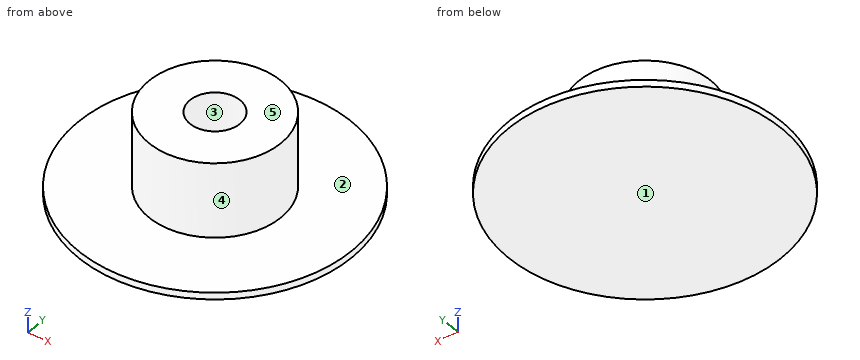
```python
from build123d import *

# Parameters (mm, degrees)
SKETCH1_R           = 30
BOSS_EXTRUDE1_DEPTH = 1.5
SKETCH2_R           = 14.5
SKETCH2_R_2         = 5.5
EXTRUDE_THIN1_DEPTH = 18


with BuildPart() as part:
    # Sketch1 → Boss-Extrude1 (new body)
    with BuildSketch(Plane.XY):
        Circle(SKETCH1_R)
    extrude(amount=BOSS_EXTRUDE1_DEPTH)

    # Sketch2 → Extrude-Thin1 (add)
    with BuildSketch(Plane.XY):
        Circle(SKETCH2_R)
        Circle(SKETCH2_R_2, mode=Mode.SUBTRACT)
    extrude(amount=EXTRUDE_THIN1_DEPTH)


solid = part.part
```
Verification items for the finished model (mm, model axes). Face numbers are marked on the shaded views. A direction names the side the tool comes from. Coordinates: 2 decimals unless noted, no trailing zeros. Loops run counter-clockwise (first coordinate to the right, second up) from the corner with the lowest first, then second, coordinate; pieces in that order, holes last. Notation, with made-up numbers: (-3, 25) -> (41, 25) arc R26 ccw to (41, 54) -> close; hole circle Ø2 at (57.5, -39). An arc over 180 degrees is marked (long way). Put each result on its own line as item: value.
1. Gauge pin test, flat ends, axial feed: P1, Ø10, axis at x = 5, z = 15.5, coming from the -Y side; P2, Ø2, axis at x = 18, y = -12.5, coming from the -Z side; P3, Ø8, axis at x = 3.5, z = 15.5, coming from the +Y side; P4, Ø1.5, axis at x = 2.5, z = 15, coming from the +Y side. Record the tip position at first contact, or that the pin passes through.
Result set:
P1: stops at y = -14.5
P2: stops at z = 0
P3: stops at y = 14.5
P4: stops at y = 14.39
2. Section check A-A, the plane y = 0. Record the boundary of the cut face in (x, z), then the cut area to 3 significant figures.
Result set:
outline: (-30, 0) -> (30, 0) -> (30, 1.5) -> (14.5, 1.5) -> (14.5, 18) -> (5.5, 18) -> (5.5, 1.5) -> (-5.5, 1.5) -> (-5.5, 18) -> (-14.5, 18) -> (-14.5, 1.5) -> (-30, 1.5) -> close
area: 387 mm^2
3. Section check C-C, the plane z = 14.25. Record the boundary of the cut face in (x, y).
Result set:
outline: circle Ø29 at (0, 0); hole circle Ø11 at (0, 0)
4. Mould release check, pull along Y, two halves, no side actions. Record for the marked faces 3, 4 and 5: pulls with the +Y half, pulls with the -Y half, needs draft (parallel to the pull), parting line crosses it, or undercut.
Result set:
face 3: undercut
face 4: parting line crosses it
face 5: needs draft
5. Thickness scan on line 1 (Y direction, x = 0, z = 5.75); line 2 (Z direction, x = -10, y = -18). Record the ranges inside material, lowest first.
Result set:
line 1: y = -14.5 to -5.5, 5.5 to 14.5
line 2: z = 0 to 1.5
6. Tool access check on the marked faces 1 and 2. Record the directions out of +Z, -Z, +X, -X, +Y, -Y that give a thin tool (end or side, any length) a straight path to the whole face; none if there is none.
Result set:
face 1: -Z, +X, -X, +Y, -Y
face 2: +Z
7. Section check D-D, the plane y = -8.5. Record the boundary of the cut face in (x, z), then the cut area to 3 significant figures.
Result set:
outline: (-28.77, 0) -> (28.77, 0) -> (28.77, 1.5) -> (11.75, 1.5) -> (11.75, 18) -> (-11.75, 18) -> (-11.75, 1.5) -> (-28.77, 1.5) -> close
area: 474 mm^2
